Source: three-view drawing plus pictorial views. Frame: mm from the lowest corner of the part. Round coordinates to 2 decimals unless told otherwise and drop trailing zeros. Write each loop counter-clockwise with the first axis right and the second up, starting at its lowest first coordinate (ties: lowest second). Pieces come first, ordered by that corner, then holes. Notation, with made-up numbers: (49.25, 34) -> (80.25, 34) arc R18 ccw to (80.25, 42) -> close; hole circle Ø2 at (-28, -38). An arc over 180 degrees is marked (long way). Put each result on its own line as item: value.
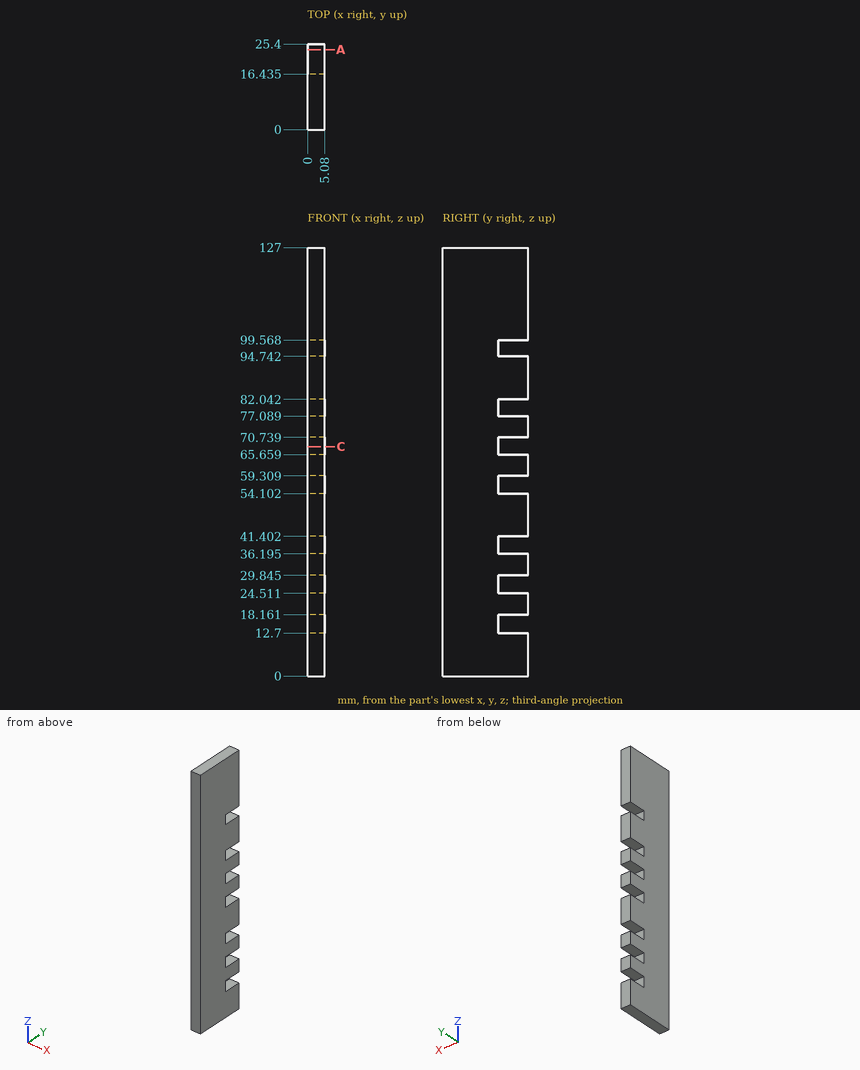
Q1. Cut plane C-C on z = 68. Output: boundary loops of the cut face in (x, y) (1 decimal).
Ans:
outline: (0, 0) -> (5.1, 0) -> (5.1, 16.4) -> (0, 16.4) -> close
Q2. Cut plane A-A on y = 23.75. Give the number of separate pieces and of enclosed holes in the cut face, and give its area (3 significant figures).
Ans:
separate pieces: 8
enclosed holes: 0
area: 462 mm^2
Q3. Pin query (flat end, axial travel): pin 1 (2.5 mm diameter, centred on x = 3, z = 38, fed in from +Y) (1 decimal). Return the tip coordinate at first contact, or that it passes through.
Ans:
pin 1: stops at y = 16.4
Q4. Material intervals for line 1 (Y direction, x = 2.4, z = 16) (1 decimal), sorted ascending. Write a range as [from, to].
Ans:
line 1: y = [0, 16.4]
